Could you check a few things on this model? Use its own coordinates, in mm. A direction names the side the tool comes from. Give positions to 0.01 mm unless a question says otherwise; leave off trailing zeros. Loops run counter-clockwise (first coordinate to the right, second up) from the corner with the lowest first, then second, coordinate; pieces in that order, holes last. Notation, with made-up numbers: M -11,56.5 L 11,56.5 A18 cw 11,79.5 Z; hole C -21,75 d8. An arc over 180 degrees is marked long. Return JSON: item names as keys, results as strings. Group by question number.
1. If we section it at D-D (z = -7): Write out the boundary of the cut face in (x, y), plus the area to 3 significant figures.
2. If we mould it in two halves opening along X, with no side actions, what happens to faces 4 (the flat face through (34.8, 1.5, -17)), 5 (the cylindrical face through (4.166, 1.254, -26.522)), 6 (the flat face through (17, 0, -17))? For each: +X half, -X half, draft (parallel to the pull), parting line (faces both ways), or undercut.
3. If we section it at C-C (x = 3.7): Write out the boundary of the cut face in (y, z).
4. If we section it at B-B (z = -19): Write out the boundary of the cut face in (x, y).
5. If we section it at A-A (y = 3.5): Write out the boundary of the cut face in (x, z), plus the area to 3 significant figures.
6. For pin 1 (1 mm diameter, centred on x = 22, z = -29.5, fed in from +Y); pin 2 (6 mm diameter, centred on x = 17, z = -22.5, fed in from +Y); pin 3 (6 mm diameter, centred on y = 7.5, z = -12, fed in from -X), each with a flat end and sliding along its axis, tell me the tip position at first contact or that it passes through.
7. Please list where these lines run through material, in increasing order: line 1 (X direction, y = 9.25, z = -27.1); line 2 (X direction, y = 1.45, z = -28); line 3 (Y direction, x = 6, z = -18).
8. For faces 1 (the flat face through (21.694, 11.748, -26.57)), 2 (the flat face through (4, 1, -28)), 3 (the cylindrical face through (17.6, 6.3, -30.2)), which set-ups out of +Z, -Z, +X, -X, +Y, -Y let a thin tool reach every point of the face, with its end or its side?
```python
from build123d import *

# Parameters (mm, degrees)
SKETCH1_W           = 35.3
SKETCH1_H           = 34.42
BOSS_EXTRUDE1_DEPTH = 2
BOSS_EXTRUDE2_DEPTH = 8.8
SKETCH4_R           = 1.55
CUT_EXTRUDE2_DEPTH  = 1
CHAMFER4_SIZE       = 0.5
BOSS_EXTRUDE3_DEPTH = 1.25
SKETCH7_R           = 1.7
CUT_EXTRUDE6_DEPTH  = 51.472432079
SKETCH6_R           = 2.85
CUT_EXTRUDE5_DEPTH  = 3
CHAMFER5_SIZE       = 0.5
CHAMFER3_SIZE       = 1
CHAMFER6_SIZE       = 0.4


with BuildPart() as part:
    # Sketch1 → Boss-Extrude1 (new body)
    with BuildSketch(Plane(origin=(0, 0, 0), x_dir=(1, 0, 0), z_dir=(0, 1, 0))):
        with Locations((17.65, 17.21)):
            Rectangle(SKETCH1_W, SKETCH1_H)
    extrude(amount=BOSS_EXTRUDE1_DEPTH)

    # Sketch2 → Boss-Extrude2 (add)
    with BuildSketch(Plane(origin=(0, 2, 0), x_dir=(1, 0, 0), z_dir=(0, 1, 0))):
        with BuildLine():
            Line((11.45, 28), (14.683520605, 28))
            ThreePointArc((14.683520605, 28), (17.65, 30.2), (20.616479395, 28))
            Line((20.616479395, 28), (23.85, 28))
            Line((23.85, 28), (23.85, 10))
            Line((23.85, 10), (11.45, 10))
            Line((11.45, 10), (11.45, 28))
        make_face()
    extrude(amount=BOSS_EXTRUDE2_DEPTH)

    # Sketch4 → Cut-Extrude2 (cut)
    with BuildSketch(Plane(origin=(0, 2, 0), x_dir=(1, 0, 0), z_dir=(0, 1, 0))):
        with Locations(Location((3.7, 28, 0), (0, 0, 270))):
            Circle(SKETCH4_R)
        with Locations(Location((31.6, 28, 0), (0, 0, 90))):
            Circle(SKETCH4_R)
    extrude(amount=-CUT_EXTRUDE2_DEPTH, mode=Mode.SUBTRACT)

    # Chamfer4
    chamfer4_edges = [part.edges().sort_by_distance(p)[0] for p in [
        (3.7, 2, -29.55),
        (31.6, 2, -26.45),
    ]]
    chamfer(chamfer4_edges, length=CHAMFER4_SIZE)

    # Sketch3 → Boss-Extrude3 (add)
    with BuildSketch(Plane(origin=(0, 10.8, 0), x_dir=(1, 0, 0), z_dir=(0, 1, 0))):
        Polygon((14.573402303, 28), (13.011701152, 25), (11.45, 28), align=None)
        Polygon((23.85, 28), (22.288298848, 25), (20.726597697, 28), align=None)
    extrude(amount=BOSS_EXTRUDE3_DEPTH)

    # Sketch7 → Cut-Extrude6 (cut, through all)
    with BuildSketch(Plane(origin=(0, 10.8, 0), x_dir=(1, 0, 0), z_dir=(0, 1, 0))):
        with Locations(Location((17.65, 27.1, 0), (0, 0, 270))):
            Circle(SKETCH7_R)
    extrude(amount=-CUT_EXTRUDE6_DEPTH, mode=Mode.SUBTRACT)

    # Sketch6 → Cut-Extrude5 (cut)
    with BuildSketch(Plane.XZ):
        with Locations(Location((17.65, -27.1, 0), (0, 0, 270))):
            Circle(SKETCH6_R)
    extrude(amount=-CUT_EXTRUDE5_DEPTH, mode=Mode.SUBTRACT)

    # Chamfer5
    chamfer5_edges = [part.edges().sort_by_distance(p)[0] for p in [
        (22.288298848, 12.05, -28),
        (21.507448273, 12.05, -26.5),
        (23.069149424, 12.05, -26.5),
        (13.011701152, 12.05, -28),
        (12.230850576, 12.05, -26.5),
        (13.792551727, 12.05, -26.5),
    ]]
    chamfer(chamfer5_edges, length=CHAMFER5_SIZE)

    # Chamfer3
    chamfer3_edges = [part.edges().sort_by_distance(p)[0] for p in [
        (35.3, 2, -17.21),
        (17.65, 2, -34.42),
        (0, 2, -17.21),
    ]]
    chamfer(chamfer3_edges, length=CHAMFER3_SIZE)

    # Chamfer6
    chamfer6_edges = [part.edges().sort_by_distance(p)[0] for p in [
        (17.65, 0, -34.42),
    ]]
    chamfer(chamfer6_edges, length=CHAMFER6_SIZE)


solid = part.part
```
Answer:
{
 "1": {"outline": "M 0,0 L 35.3,0 L 35.3,1 L 34.3,2 L 1,2 L 0,1 Z", "area": "69.6 mm²"},
 "2": {"face 4": "+X half", "face 5": "undercut", "face 6": "draft"},
 "3": {"outline": "M 0,-34.02 L 0.4,-34.42 L 1,-34.42 L 2,-33.42 L 2,-30.05 L 1.5,-29.55 L 1,-29.55 L 1,-26.45 L 1.5,-26.45 L 2,-25.95 L 2,0 L 0,0 Z"},
 "4": {"outline": "M 0,0 L 35.3,0 L 35.3,1 L 34.3,2 L 23.85,2 L 23.85,10.8 L 11.45,10.8 L 11.45,2 L 1,2 L 0,1 Z"},
 "5": {"outline": "M 11.45,-28 L 14.68,-28 A3.1 ccw 20.62,-28 L 23.85,-28 L 23.85,-10 L 11.45,-10 Z; hole C 17.65,-27.1 d3.4", "area": "224 mm²"},
 "6": {"pin 1": "stops at y = 2", "pin 2": "stops at y = 10.8", "pin 3": "stops at x = 11.45"},
 "7": {"line 1": "x = 11.45 to 15.95, 19.35 to 23.85", "line 2": "x = 0.45 to 2.15, 5.25 to 14.95, 20.35 to 30.05, 33.15 to 34.85", "line 3": "y = 0 to 2"},
 "8": {"face 1": "+Z, +Y", "face 2": "+Y", "face 3": "-Z, +Y"}
}
